```python
from build123d import *

# Parameters (mm, degrees)
SKETCH1_R           = 2.286
BOSS_EXTRUDE1_DEPTH = 3.175
FILLET1_R           = 6.35


with BuildPart() as part:
    # Sketch1 → Boss-Extrude1 (new body)
    with BuildSketch(Plane.XY):
        with BuildLine():
            Line((-11.14552, -8.494944846), (1.143, -6.246282975))
            ThreePointArc((1.143, -6.246282975), (4.87752755, -4.065983891), (6.35, 0))
            Line((6.35, 0), (6.35, 63.5))
            ThreePointArc((6.35, 63.5), (3.763735435, 68.614371474), (-1.88836081, 69.562721621))
            Line((-1.88836081, 69.562721621), (-15.268170702, 65.395301404))
            ThreePointArc((-15.268170702, 65.395301404), (-21.178428452, 58.792177512), (-18.161, 50.459859867))
            Line((-18.161, 50.459859867), (-18.161, 6.690140133))
            ThreePointArc((-18.161, 6.690140133), (-20.53976569, -3.621956643), (-11.14552, -8.494944846))
        make_face()
        Circle(SKETCH1_R, mode=Mode.SUBTRACT)
        with Locations((0, 63.5)):
            Circle(SKETCH1_R, mode=Mode.SUBTRACT)
        with BuildLine():
            Line((-14.986, 0), (-14.986, 57.15))
            ThreePointArc((-14.986, 57.15), (-12.7, 59.436), (-10.414, 57.15))
            Line((-10.414, 57.15), (-10.414, 0))
            ThreePointArc((-10.414, 0), (-12.7, -2.286), (-14.986, 0))
        make_face(mode=Mode.SUBTRACT)
    extrude(amount=BOSS_EXTRUDE1_DEPTH)

    # Fillet1
    fillet1_edges = [part.edges().sort_by_distance(p)[0] for p in [
        (-18.161, 6.690140133, 1.5875),
        (-18.161, 50.459859867, 1.5875),
    ]]
    fillet(fillet1_edges, radius=FILLET1_R)


solid = part.part
```
CAD build for the part. Positions are in the model's coordinates, mm. A direction names the side the tool comes from. Coordinates: 2 decimals unless noted, no trailing zeros. Loops run counter-clockwise (first coordinate to the right, second up) from the corner with the lowest first, then second, coordinate; pieces in that order, holes last. Notation, with made-up numbers: (52.25, -40) - (95.25, -40) arc R18 cw to (95.25, -5) - close; hole circle Ø5 at (72.5, 31). An arc over 180 degrees is marked (long way). Return JSON: item names as keys, results as strings.
1. Probe L1, parallel to X at y = 20, z = 1.2; L2, parallel to Y at x = 2, z = 1.65; L3, parallel to Y at x = 0, z = 0.8. List the from-to ranges inside material, lowest first. Write a range as from..to.
Result:
{"L1": "x = -18.16..-14.99, -10.41..6.35", "L2": "y = -6.03..-1.11, 1.11..62.39, 64.61..69.53", "L3": "y = -6.46..-2.29, 2.29..61.21, 65.79..69.85"}
2. Band-saw the part on B-B (x = -12.7). Give the cut face in (y, z) (3 decimals), and give its area (3 significant figures).
Result:
{"outline": "(-8.636, 0) - (-2.286, 0) - (-2.286, 3.175) - (-8.636, 3.175) - close; (59.436, 0) - (66.195, 0) - (66.195, 3.175) - (59.436, 3.175) - close", "area": "41.6 mm2"}
3. Band-saw the part on A-A (y = 46). Give the cut face in (x, z) (3 decimals), and give its area (3 significant figures).
Result:
{"outline": "(-18.161, 0) - (-14.986, 0) - (-14.986, 3.175) - (-18.161, 3.175) - close; (-10.414, 0) - (6.35, 0) - (6.35, 3.175) - (-10.414, 3.175) - close", "area": "63.3 mm2"}
4. Band-saw the part on D-D (x = 0). Give the cut face in (y, z) (3 decimals).
Result:
{"outline": "(-6.455, 0) - (-2.286, 0) - (-2.286, 3.175) - (-6.455, 3.175) - close; (2.286, 0) - (61.214, 0) - (61.214, 3.175) - (2.286, 3.175) - close; (65.786, 0) - (69.85, 0) - (69.85, 3.175) - (65.786, 3.175) - close"}
5. Mould opens along X. For faces 1 (the flat face through (-18.161, 29, 2)), 2 (the cylindrical face through (-12.75, 59.435, 1.565)), 3 (the flat face through (6.35, 31, 2)) say: released by +X, released by -X, zero draft, split by the parting line, or undercut.
Result:
{"face 1": "released by -X", "face 2": "undercut", "face 3": "released by +X"}
6. Drop a flat-ended pin along its axis: pin 1 (1.6 mm diameter, centred on y = 17, z = 2, fed in from -X). Give the stop position or say it passes through.
Result:
{"pin 1": "stops at x = -18.16"}
7. Band-saw the part on C-C (z = 0.8). Give the cut face in (x, y).
Result:
{"outline": "(-19.51, 5.32) arc R8.64 ccw to (-11.15, -8.49) - (1.14, -6.25) arc R6.35 ccw to (6.35, 0) - (6.35, 63.5) arc R6.35 ccw to (-1.89, 69.56) - (-15.27, 65.4) arc R8.64 ccw to (-19.51, 51.83) arc R6.35 cw to (-18.16, 47.93) - (-18.16, 9.22) arc R6.35 cw to start; hole (-14.99, 0) arc R2.29 ccw to (-10.41, 0) - (-10.41, 57.15) arc R2.29 ccw to (-14.99, 57.15) - close; hole circle Ø4.57 at (0, 0); hole circle Ø4.57 at (0, 63.5)"}
8. 3-axis set-ups, long thin cutter, end or side, ignore diameter. For faces 4 (the cylindrical face through (-12.65, -2.285, 1.565)), 5 (the cylindrical face through (-18.516, 7.129, 1.61)), 6 (the flat face through (-5, 31, 0)): which of +Z, -Z, +X, -X, +Y, -Y reach the whole face in a straight line?
Result:
{"face 4": "+Z, -Z", "face 5": "+Z, -Z, -X", "face 6": "-Z, +X, -X, +Y, -Y"}
